```python
from build123d import *

# Parameters (mm, degrees)
SKETCH1_W           = 31
SKETCH1_H           = 40
SKETCH1_W_2         = 21
SKETCH1_H_2         = 30
BOSS_EXTRUDE1_DEPTH = 2
SKETCH2_W           = 31
SKETCH2_H           = 40
SKETCH2_W_2         = 29
SKETCH2_H_2         = 34
BOSS_EXTRUDE2_DEPTH = 19
SKETCH4_W           = 5
SKETCH4_H           = 10
SKETCH4_R           = 2
BOSS_EXTRUDE3_DEPTH = 3
BOSS_EXTRUDE4_START = -21
SKETCH5_W           = 3
SKETCH5_H           = 50.481247069
BOSS_EXTRUDE4_DEPTH = 21
FILLET2_R           = 1.5
SKETCH7_W           = 6
SKETCH7_H           = 3
CUT_EXTRUDE4_DEPTH  = 2


with BuildPart() as part:
    # Sketch1 → Boss-Extrude1 (new body)
    with BuildSketch(Plane(origin=(0, 0, 0), x_dir=(1, 0, 0), z_dir=(0, 1, 0))):
        Rectangle(SKETCH1_W, SKETCH1_H)
        Rectangle(SKETCH1_W_2, SKETCH1_H_2, mode=Mode.SUBTRACT)
    extrude(amount=BOSS_EXTRUDE1_DEPTH)

    # Sketch2 → Boss-Extrude2 (add)
    with BuildSketch(Plane(origin=(0, 2, 0), x_dir=(1, 0, 0), z_dir=(0, 1, 0))):
        Rectangle(SKETCH2_W, SKETCH2_H)
        Rectangle(SKETCH2_W_2, SKETCH2_H_2, mode=Mode.SUBTRACT)
    extrude(amount=BOSS_EXTRUDE2_DEPTH)

    # Sketch4 → Boss-Extrude3 (add)
    with BuildSketch(Plane(origin=(0, 21, 0), x_dir=(1, 0, 0), z_dir=(0, 1, 0))):
        with Locations((18, -2)):
            Rectangle(SKETCH4_W, SKETCH4_H)
        with Locations(Location((17.51, -2, 0), (0, 0, 270))):
            Circle(SKETCH4_R, mode=Mode.SUBTRACT)
    boss_extrude3 = extrude(amount=-BOSS_EXTRUDE3_DEPTH)

    # Mirror1: Boss-Extrude3 across plane
    add(boss_extrude3.mirror(Plane(origin=(0, 0, 0), x_dir=(0, 0, 1), z_dir=(1, 0, 0))))

    # Sketch5 → Boss-Extrude4 (add)
    with BuildSketch(Plane.XZ.offset(BOSS_EXTRUDE4_START)):
        with Locations((0, 45.240623535)):
            Rectangle(SKETCH5_W, SKETCH5_H)
        Polygon((-41.352486375, -32.973806719), (-43.473806719, -30.852486375), (-15.5, -2.878679656), (-15.5, -7.121320344), align=None)
        Polygon((15.5, -2.878679656), (43.473806719, -30.852486375), (41.352486375, -32.973806719), (15.5, -7.121320344), align=None)
    extrude(amount=BOSS_EXTRUDE4_DEPTH)

    # Fillet2
    fillet2_edges = [part.edges().sort_by_distance(p)[0] for p in [
        (-41.352486375, 10.5, -32.973806719),
        (-43.473806719, 10.5, -30.852486375),
        (41.352486375, 10.5, -32.973806719),
        (43.473806719, 10.5, -30.852486375),
        (1.5, 10.5, 70.481247069),
        (-1.5, 10.5, 70.481247069),
        (1.5, 10.5, 20),
        (-1.5, 10.5, 20),
        (-15.5, 10.5, -7.121320344),
        (15.5, 10.5, -7.121320344),
    ]]
    fillet(fillet2_edges, radius=FILLET2_R - 0.0001)  # a hair under: the kernel refuses the full size

    # Sketch7 → Cut-Extrude4 (cut)
    with BuildSketch(Plane(origin=(0, 21, 0), x_dir=(1, 0, 0), z_dir=(0, 1, 0))):
        with Locations((0, 18.5)):
            Rectangle(SKETCH7_W, SKETCH7_H)
    extrude(amount=-CUT_EXTRUDE4_DEPTH, mode=Mode.SUBTRACT)


solid = part.part
```
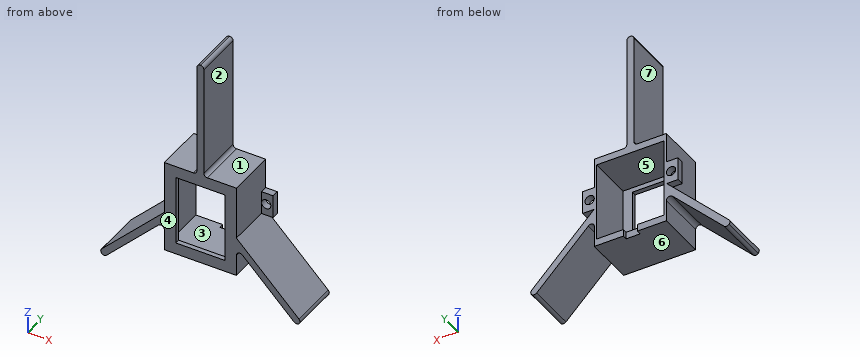
Design review of the part built by this model. Coordinates are the model's own, in mm. Face numbers are marked on the shaded views. A direction names the side the tool comes from. Round coordinates to 2 decimals unless told otherwise and drop trailing zeros. Order: outer loops, then holes, each group sorted by start corner. A loop starts at its lowest first (then second) coordinate and runs counter-clockwise, first axis right, second up. Notation, with made-up numbers: (26.5, 26.25) - (84.5, 26.25) arc R34 ccw to (84.5, 64.25) - close; hole circle Ø6 at (68.25, 86.25). An arc over 180 degrees is marked (long way). Return JSON: item names as keys, results as strings.
Q1. Consider section D-D on z = 29. Write out the cut boundary in (x, y), plus the area to 3 significant figures.
Computed values:
{"outline": "(-1.5, 0) - (1.5, 0) - (1.5, 21) - (-1.5, 21) - close", "area": "63.0 mm2"}
Q2. Consider section A-A on z = 11. Write out the cut boundary in (x, y), plus the area to 3 significant figures.
Computed values:
{"outline": "(-15.5, 0) - (-10.5, 0) - (-10.5, 2) - (-14.5, 2) - (-14.5, 21) - (-15.5, 21) - close; (10.5, 0) - (15.5, 0) - (15.5, 21) - (14.5, 21) - (14.5, 2) - (10.5, 2) - close", "area": "58.0 mm2"}
Q3. Wall thickness on L1, parallel to X at y = 20.1, z = 2; L2, parallel to Z at x = 9.5, y = 7.5; L3, parallel to X at y = 15.5, z = 1: over which ranges is each line inside the solid? List them lowest first. Write a range as [from, to].
Computed values:
{"L1": "x = [-20.5, -19.51], [-15.51, -14.5], [14.5, 15.51], [19.51, 20.5]", "L2": "z = [-20, -17], [17, 20]", "L3": "x = [-15.5, -14.5], [14.5, 15.5]"}
Q4. Consider section B-B on x = 5. Write out the cut boundary in (y, z).
Computed values:
{"outline": "(0, -20) - (21, -20) - (21, -17) - (2, -17) - (2, -15) - (0, -15) - close; (0, 15) - (2, 15) - (2, 17) - (21, 17) - (21, 20) - (0, 20) - close"}
Q5. Machinability: for the marked faces 4, 5, 6 and 7, which of the approach directions +Z, -Z, +X, -X, +Y, -Y give a long, thin tool a straight path to every point of the face, cutting with its end or side? Answer none if there is none.
Computed values:
{"face 4": "+Z, -Z, +X, -X, -Y", "face 5": "+Y", "face 6": "-Z, +Y, -Y", "face 7": "+Z, -X, +Y, -Y"}
Q6. The part is to be moulded in two halves that separate along Z. For the marked faces 1, 2 and 3, say which applies: pulls with the +Z half, pulls with the -Z half, needs draft (parallel to the pull), parting line crosses it, or undercut.
Computed values:
{"face 1": "pulls with the +Z half", "face 2": "needs draft", "face 3": "undercut"}
Q7. For pin 1 Ø0.9 at (x, z) = (-0.5, -18) entering from +Y; pin 2 Ø1.5 at (x, y) = (-7, 11.5) entering from +Z; pin 3 Ø3 at (y, z) = (13, -14) entering from -X; pin 4 Ø3.5 at (x, z) = (17.51, 2) entering from -Y, all flat-tipped, find the tip position at first contact; note any pin that passes through.
Computed values:
{"pin 1": "stops at y = 19", "pin 2": "stops at z = 20", "pin 3": "stops at x = -28.12", "pin 4": "passes through"}
